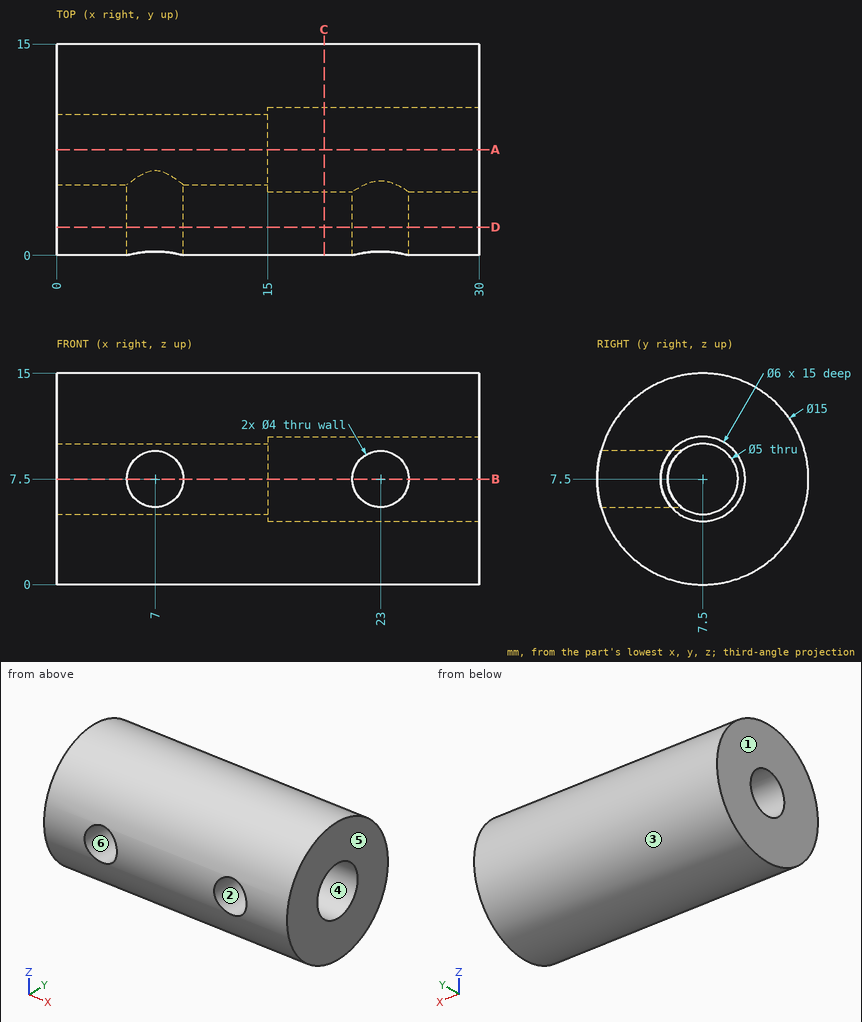
Verification items for this drawing (mm, ordinates from the low corner). A direction names the side the tool comes from. Give positions to 0.01 mm unless a question says otherwise; leave off trailing zeros. Loops run counter-clockwise (first coordinate to the right, second up) from the corner with the lowest first, then second, coordinate; pieces in that order, holes last.
1. Tool access check on the marked faces 4, 5 and 6. Record the directions out of +Z, -Z, +X, -X, +Y, -Y that give a thin tool (end or side, any length) a straight path to the whole face; none if there is none.
Derived:
face 4: +X
face 5: +Z, -Z, +X, +Y, -Y
face 6: -Y
2. Material ranges on probe 1 along X at (y, z) = (1.5, 7.5); probe 2 along Y at (x, z) = (4, 7.5); probe 3 along X at (y, z) = (1, 6), recorded low to high.
Derived:
probe 1: x = 0 to 5, 9 to 21, 25 to 30
probe 2: y = 0 to 5, 10 to 15
probe 3: x = 0 to 5.68, 8.32 to 21.68, 24.32 to 30
3. Cross-section at C-C on x = 19. Record the cut outline in (y, z), and give its area (3 significant figures).
Derived:
outline: circle Ø15 at (7.5, 7.5); hole circle Ø6 at (7.5, 7.5)
area: 148 mm2
4. Go/stop test with flat-tipped pins: P1, Ø2.5, axis at x = 23, z = 7.5, coming from the -Y side; P2, Ø1, axis at x = 25, y = 11.5, coming from the -Z side; P3, Ø6, axis at x = 26, z = 2, coming from the -Y side. Record where each tip stops, or that it passes through.
Derived:
P1: stops at y = 10.23
P2: stops at z = 0.87
P3: stops at y = 0.43
5. Cross-section at B-B on z = 7.5. Record the cut outline in (x, y).
Derived:
outline: (0, 0) - (5, 0) - (5, 5) - (0, 5) - close; (0, 10) - (15, 10) - (15, 10.5) - (30, 10.5) - (30, 15) - (0, 15) - close; (9, 0) - (21, 0) - (21, 4.5) - (15, 4.5) - (15, 5) - (9, 5) - close; (25, 0) - (30, 0) - (30, 4.5) - (25, 4.5) - close
6. Cross-section at A-A on y = 7.5. Record the cut outline in (x, z), and give its area (3 significant figures).
Derived:
outline: (0, 0) - (30, 0) - (30, 4.5) - (15, 4.5) - (15, 5) - (0, 5) - close; (0, 10) - (15, 10) - (15, 10.5) - (30, 10.5) - (30, 15) - (0, 15) - close
area: 285 mm2
7. Release check for a two-part mould opening along Z. For the marked faces 1, 2 and 3 record: +Z half, -Z half, draft (parallel to the pull), parting line (faces both ways), or undercut.
Derived:
face 1: draft
face 2: undercut
face 3: parting line
8. Cross-section at D-D on y = 2. Record the cut outline in (x, z), and give its area (3 significant figures).
Derived:
outline: (0, 2.4) - (30, 2.4) - (30, 12.6) - (0, 12.6) - close; hole circle Ø4 at (7, 7.5); hole circle Ø4 at (23, 7.5)
area: 281 mm2
